from build123d import *

# Parameters (mm, degrees)
BOSS_EXTRUDE1_DEPTH = 3.175
CUT_EXTRUDE1_REACH  = 53.782
SKETCH2_R           = 11
CUT_EXTRUDE2_REACH  = 53.782
SKETCH3_W           = 25.4
SKETCH3_H           = 5.715
CUT_EXTRUDE4_REACH  = 53.782
SKETCH6_R           = 1.3250037
CUT_EXTRUDE6_DEPTH  = 52.781708168
SKETCH7_R           = 10
CUT_EXTRUDE7_DEPTH  = 52.781708168
FILLET1_R           = 6.35
CUT_EXTRUDE8_REACH  = 53.782
SKETCH8_W           = 6.604
SKETCH8_H           = 10.16


with BuildPart() as part:
    # Sketch1 → Boss-Extrude1 (new body)
    with BuildSketch(Plane.XY):
        with BuildLine():
            Line((30.48, -11.260079969), (-30.48, -11.260079969))
            Line((-30.48, -11.260079969), (-30.48, 11.260079969))
            ThreePointArc((-30.48, 11.260079969), (0, 41.740079969), (30.48, 11.260079969))
            Line((30.48, 11.260079969), (30.48, -11.260079969))
        make_face()
    extrude(amount=BOSS_EXTRUDE1_DEPTH)

    # Sketch2 → Cut-Extrude1 (cut, up to next)
    with BuildSketch(Plane.XY.offset(3.175), mode=Mode.PRIVATE) as cut_extrude1_sk1:
        with Locations((0, 19.504919969)):
            Circle(SKETCH2_R)
    cut_extrude1_tool1 = extrude(cut_extrude1_sk1.sketch, amount=-CUT_EXTRUDE1_REACH, mode=Mode.PRIVATE) & part.part
    add(cut_extrude1_tool1.solids().sort_by_distance((0, 19.50492, 3.175))[0], mode=Mode.SUBTRACT)

    # Sketch3 → Cut-Extrude2 (cut, up to next)
    with BuildSketch(Plane.XY.offset(3.175), mode=Mode.PRIVATE) as cut_extrude2_sk1:
        with Locations((0, -8.402579969)):
            Rectangle(SKETCH3_W, SKETCH3_H)
    cut_extrude2_tool1 = extrude(cut_extrude2_sk1.sketch, amount=-CUT_EXTRUDE2_REACH, mode=Mode.PRIVATE) & part.part
    add(cut_extrude2_tool1.solids().sort_by_distance((0, -8.40258, 3.175))[0], mode=Mode.SUBTRACT)

    # Sketch5 → Cut-Extrude4 (cut, up to next)
    with BuildSketch(Plane.XY.offset(3.175), mode=Mode.PRIVATE) as cut_extrude4_sk1:
        Polygon((3.175, -1.735079969), (1.143, -1.735079969), (1.143, -5.545079969), (-1.143, -5.545079969), (-1.143, -1.735079969), (-3.175, -1.735079969), (-3.175, 0.804920031), (-1.143, 0.804920031), (-1.143, 9.694920031), (1.143, 9.694920031), (1.143, 0.804920031), (3.175, 0.804920031), align=None)
    cut_extrude4_tool1 = extrude(cut_extrude4_sk1.sketch, amount=-CUT_EXTRUDE4_REACH, mode=Mode.PRIVATE) & part.part
    add(cut_extrude4_tool1.solids().sort_by_distance((0, 1.494349, 3.175))[0], mode=Mode.SUBTRACT)

    # Sketch6 → Cut-Extrude6 (cut, through all)
    with BuildSketch(Plane.XY):
        with Locations((0, 33.004919969)):
            Circle(SKETCH6_R)
        with Locations((11.691342951, 12.754919969)):
            Circle(SKETCH6_R)
        with Locations((-11.691342951, 12.754919969)):
            Circle(SKETCH6_R)
    extrude(amount=CUT_EXTRUDE6_DEPTH, mode=Mode.SUBTRACT)

    # Sketch7 → Cut-Extrude7 (cut, through all)
    with BuildSketch(Plane.XY):
        with Locations((0, 13.504920031)):
            Circle(SKETCH7_R)
    extrude(amount=CUT_EXTRUDE7_DEPTH, mode=Mode.SUBTRACT)

    # Fillet1
    fillet1_edges = [part.edges().sort_by_distance(p)[0] for p in [
        (9.921567423, 14.754919982, 1.5875),
        (-9.921567423, 14.754919982, 1.5875),
    ]]
    fillet(fillet1_edges, radius=FILLET1_R)

    # Sketch8 → Cut-Extrude8 (cut, up to next)
    with BuildSketch(Plane.XY.offset(3.175), mode=Mode.PRIVATE) as cut_extrude8_sk1:
        with Locations((22.86, 6.519920031)):
            Rectangle(SKETCH8_W, SKETCH8_H)
    cut_extrude8_tool1 = extrude(cut_extrude8_sk1.sketch, amount=-CUT_EXTRUDE8_REACH, mode=Mode.PRIVATE) & part.part
    # Sketch8 → Cut-Extrude8 (cut, up to next)
    with BuildSketch(Plane.XY.offset(3.175), mode=Mode.PRIVATE) as cut_extrude8_sk2:
        with Locations((-22.86, 6.519920031)):
            Rectangle(SKETCH8_W, SKETCH8_H)
    cut_extrude8_tool2 = extrude(cut_extrude8_sk2.sketch, amount=-CUT_EXTRUDE8_REACH, mode=Mode.PRIVATE) & part.part
    add(cut_extrude8_tool1.solids().sort_by_distance((22.86, 6.51992, 3.175))[0], mode=Mode.SUBTRACT)
    add(cut_extrude8_tool2.solids().sort_by_distance((-22.86, 6.51992, 3.175))[0], mode=Mode.SUBTRACT)


solid = part.part
Design review of the part built by this model. Coordinates are the model's own, in mm. A direction names the side the tool comes from. Coordinates: 2 decimals unless noted, no trailing zeros. Order: outer loops, then holes, each group sorted by start corner. A loop starts at its lowest first (then second) coordinate and runs counter-clockwise, first axis right, second up.
Item 1: Take a section at D-D, the plane z = 1.25. Count the separate pieces of the cut face and the enclosed holes in it, then the cut area to 3 significant figures.
Item 2: Take a section at A-A, the plane x = 0. Write out the cut boundary in (y, z) (3 decimals).
Item 3: For line 1 (X direction, y = -4.5, z = 2.4); line 2 (X direction, y = -9, z = 2.5); line 3 (X direction, y = 6.5, z = 1), list the stretches that pass through material, from the lowest coordinate up.
Item 4: Take a section at B-B, the plane y = 10. Write out the cut boundary in (x, z) (3 decimals), then the cut area to 3 significant figures.
Item 5: The part is to be moulded in two halves that separate along X. For faces 1 (the flat face through (7, 4, 0)), 2 (the flat face through (30.48, 0, 2)), 3 (the flat face through (3.175, 0, 2)), say which applies: pulls with the +X half, pulls with the -X half, needs draft (parallel to the pull), parting line crosses it, or undercut.
Item 6: For faces 4 (the flat face through (26.162, 6, 2)), 5 (the flat face through (7, -5.545, 2)), 6 (the flat face through (-21, -11.26, 2)), list the 3-axis set-ups (+Z, -Z, +X, -X, +Y, -Y) from which the entire face can be reached by the end or side of a thin tool; tool diameter is ignored.
Item 7: For pin 1 Ø1 at (x, z) = (2, 2) entering from +Y; pin 2 Ø4 at (x, y) = (21, 31) entering from -Z; pin 3 Ø1.6 at (x, z) = (-24, 2) entering from +Y; pin 4 Ø1 at (y, z) = (28, 2.5) entering from +X, all flat-tipped, find the tip position at first contact; note any pin that passes through.
Item 8: Take a section at C-C, the plane y = 21.5. Write out the cut boundary in (x, z) (3 decimals).
The answers:
1. separate pieces: 1
1. enclosed holes: 5
1. area: 2,030 mm2
2. outline: (30.505, 0) - (31.68, 0) - (31.68, 3.175) - (30.505, 3.175) - close; (34.33, 0) - (41.74, 0) - (41.74, 3.175) - (34.33, 3.175) - close
3. line 1: x = -30.48 to -1.14, 1.14 to 30.48
3. line 2: x = -30.48 to -12.7, 12.7 to 30.48
3. line 3: x = -30.48 to -26.16, -19.56 to -7.14, 7.14 to 19.56, 26.16 to 30.48
4. outline: (-30.48, 0) - (-26.162, 0) - (-26.162, 3.175) - (-30.48, 3.175) - close; (-19.558, 0) - (-9.366, 0) - (-9.366, 3.175) - (-19.558, 3.175) - close; (9.366, 0) - (19.558, 0) - (19.558, 3.175) - (9.366, 3.175) - close; (26.162, 0) - (30.48, 0) - (30.48, 3.175) - (26.162, 3.175) - close
4. area: 92.1 mm2
5. face 1: needs draft
5. face 2: pulls with the +X half
5. face 3: undercut
6. face 4: +Z, -Z
6. face 5: +Z, -Z, -Y
6. face 6: +Z, -Z, +X, -X, -Y
7. pin 1: stops at y = 41.7
7. pin 2: stops at z = 0
7. pin 3: stops at y = 31.03
7. pin 4: stops at x = 25.79
8. outline: (-28.708, 0) - (-10.818, 0) - (-10.818, 3.175) - (-28.708, 3.175) - close; (10.818, 0) - (28.708, 0) - (28.708, 3.175) - (10.818, 3.175) - close
